Geometry check sheet. Reference: drawing and pictorial views, mm from the part's lowest x, y, z. Give positions to 0.01 mm unless a question says otherwise; leave off trailing zeros. Order: outer loops, then holes, each group sorted by start corner. A loop starts at its lowest first (then second) coordinate and runs counter-clockwise, first axis right, second up. Notation, with made-up numbers: (30.5, -5.5) - (52.5, -5.5) arc R17 cw to (52.5, 5.5) - close; hole circle Ø8 at (-26, 89.5). An arc over 180 degrees is marked (long way). Answer in a Markdown table with one row per item.
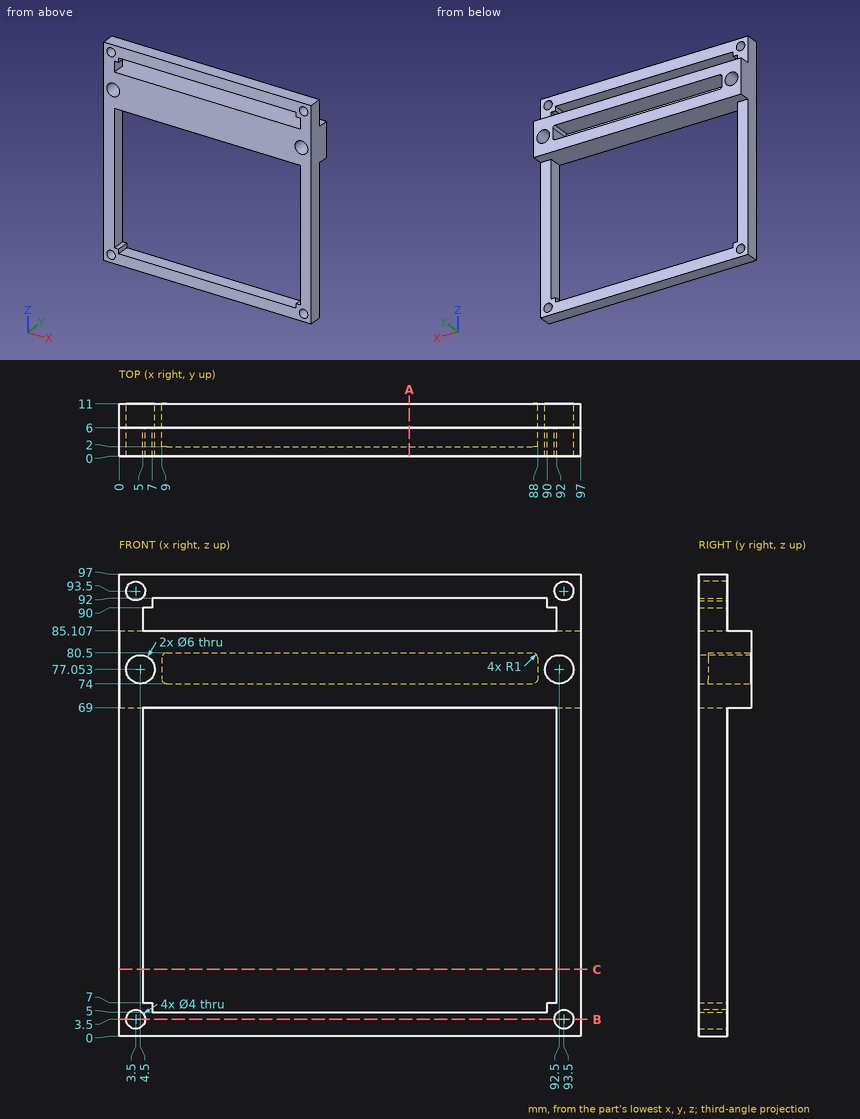
(1) Thickness scan on L1, parallel to Z at x = 62, y = 2.5; L2, parallel to X at y = 4.35, z = 3.5; L3, parallel to Z at x = 21, y = 1.5. Record the ranges inside material, lowest first.
Geometry says:
| item | result |
|---|---|
| L1 | 0 to 5, 69 to 74, 80.5 to 85.11, 92 to 97 |
| L2 | 0 to 1.5, 5.5 to 91.5, 95.5 to 97 |
| L3 | 0 to 5, 69 to 85.11, 92 to 97 |
(2) Cross-section at C-C, the plane z = 14. Record the cut outline in (x, y).
Geometry says:
| item | result |
|---|---|
| outline | (0, 0) - (5, 0) - (5, 6) - (0, 6) - close; (92, 0) - (97, 0) - (97, 6) - (92, 6) - close |
(3) Cross-section at B-B, the plane z = 3.5. Record the cut outline in (x, y).
Geometry says:
| item | result |
|---|---|
| outline | (0, 0) - (1.5, 0) - (1.5, 6) - (0, 6) - close; (5.5, 0) - (91.5, 0) - (91.5, 6) - (5.5, 6) - close; (95.5, 0) - (97, 0) - (97, 6) - (95.5, 6) - close |
(4) Cross-section at A-A, the plane x = 61. Record the cut outline in (y, z), then the cut area to 3 significant figures.
Geometry says:
| item | result |
|---|---|
| outline | (0, 0) - (6, 0) - (6, 5) - (0, 5) - close; (0, 69) - (11, 69) - (11, 74) - (2, 74) - (2, 80.5) - (11, 80.5) - (11, 85.11) - (0, 85.11) - close; (0, 92) - (6, 92) - (6, 97) - (0, 97) - close |
| area | 179 mm² |
(5) Gauge pin test, flat ends, axial feed: P1, Ø5, axis at x = 4.5, z = 77.05, coming from the +Y side; P2, Ø3, axis at x = 38.5, z = 78, coming from the +Y side. Record the tip position at first contact, or that the pin passes through.
Geometry says:
| item | result |
|---|---|
| P1 | through |
| P2 | y = 2 |
